CAD build for the part. Positions are in the model's coordinates, mm. Face numbers are marked on the shaded views. Give positions to 0.01 mm unless a question says otherwise; leave off trailing zeros. Write each loop counter-clockwise with the first axis right and the second up, starting at its lowest first coordinate (ties: lowest second). Pieces come first, ordered by that corner, then holes. Notation, with made-up numbers: (78, 66.5) - (128, 66.5) arc R12 ccw to (128, 77.5) - close; hole circle Ø10 at (-9, -6.5). An arc over 180 degrees is marked (long way). Answer as a JSON object with one key per item and string values.
Autodesk Inventor part; units mm, degrees
ref_plane "YZ Plane" through (0, 0, 0) normal (1, 0, 0) x (0, 1, 0)
ref_plane "XZ Plane" through (0, 0, 0) normal (0, 1, 0) x (-1, 0, 0)
ref_plane "XY Plane" through (0, 0, 0) normal (0, 0, 1) x (1, 0, 0)
sketch "Sketch1" plane through (0, 0, 0) normal (0, 1, 0) x (-1, 0, 0)
  circle A0 centre (0, 0) radius 2.5
  dimension "d0" = 5
extrude "Extrusion1" add sketch "Sketch1" along normal blind 58
sketch "Sketch2" plane through (0, 0, 0) normal (0, -1, 0) x (1, 0, 0)
  circle A0 centre (0, 0) radius 3.5
  dimension "d3" = 7
extrude "Extrusion2" add sketch "Sketch2" along normal blind 3
thread "Thread1"
sketch "Sketch3" plane through (0, -3, 0) normal (0, -1, 0) x (1, 0, 0)
  circle A0 centre (0, 0) radius 2.5
  line L0 (1.7236, -1.0145) -> (-0.0168, -1.9999)
  line L1 (-0.0168, -1.9999) -> (-1.7404, -0.9854)
  line L2 (-1.7404, -0.9854) -> (-1.7236, 1.0145)
  line L3 (-1.7236, 1.0145) -> (0.0168, 1.9999)
  line L4 (0.0168, 1.9999) -> (1.7404, 0.9854)
  line L5 (1.7404, 0.9854) -> (1.7236, -1.0145)
extrude "Extrusion3" cut sketch "Sketch3" against normal blind 1 contours L0 L1 L2 L3 L4 L5
properties part number "Connector_1" material "Steel, Mild"
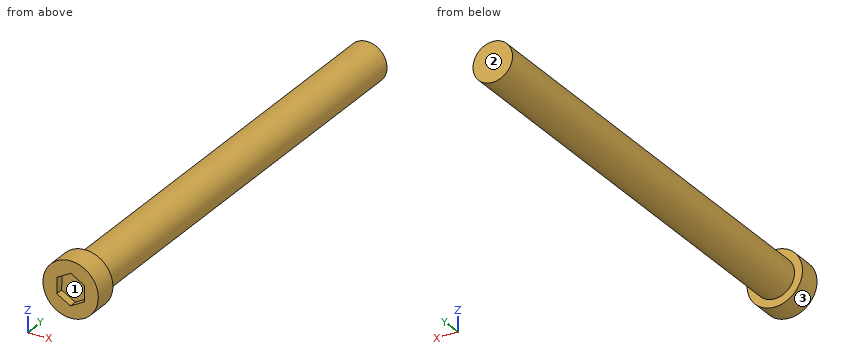
(1) Saw through at B-B, the plane x = 1. Give the cut face in (y, z).
Answer key:
{"outline": "(-3, -3.35) - (0, -3.35) - (0, -2.29) - (58, -2.29) - (58, 2.29) - (0, 2.29) - (0, 3.35) - (-3, 3.35) - (-3, 1.42) - (-2, 1.42) - (-2, -1.42) - (-3, -1.42) - close"}
(2) Saw through at A-A, the plane z = 0. Give the cut face in (x, y).
Answer key:
{"outline": "(-3.5, -3) - (-1.73, -3) - (-1.73, -2) - (1.73, -2) - (1.73, -3) - (3.5, -3) - (3.5, 0) - (2.5, 0) - (2.5, 58) - (-2.5, 58) - (-2.5, 0) - (-3.5, 0) - close"}
(3) Flat gauge pins, fed straight in: P1, Ø4, axis at x = 1, z = -2.5, coming from the +Y side; P2, Ø1, axis at x = 0, z = 0, coming from the -Y side; P3, Ø4, axis at y = 25.5, z = 1, coming from the +X side. Where does each tip first touch, or does it go through?
Answer key:
{"P1": "stops at y = 58", "P2": "stops at y = -2", "P3": "stops at x = 2.5"}
(4) Probe L1, parallel to Z at x = -1.5, y = 53.5; L2, parallel to X at y = 41.5, z = -0.25; L3, parallel to Y at x = 0.5, z = 1.5. List the from-to ranges inside material, lowest first. Write a range as [from, to].
Answer key:
{"L1": "z = [-2, 2]", "L2": "x = [-2.49, 2.49]", "L3": "y = [-2, 58]"}
(5) Saw through at C-C, the plane y = 34. Give the cut face in (x, z), and give its area (3 significant figures).
Answer key:
{"outline": "circle Ø5 at (0, 0)", "area": "19.6 mm²"}
(6) Pull direction X, two halves, no side cores. Call the marked faces 1, 2 and 3: pulls with the +X half, pulls with the -X half, needs draft (parallel to the pull), parting line crosses it, or undercut.
Answer key:
{"face 1": "undercut", "face 2": "needs draft", "face 3": "parting line crosses it"}
